Model file for the job. Use its own axes, mm. Face numbers are marked on the shaded views. A direction names the side the tool comes from. Coordinates: 2 decimals unless noted, no trailing zeros. Write each loop counter-clockwise with the first axis right and the second up, starting at its lowest first coordinate (ties: lowest second). Pieces come first, ordered by that corner, then holes. Notation, with made-up numbers: M 13.5,64.25 L 35.5,64.25 A18 ccw 35.5,96.25 Z; hole C 40,-12.5 d2. An arc over 180 degrees is marked long. One line per question, with ' | ' between items. Start each with the question number.
(1) Cut at A-A (y = -35). Write the cut outline in (x, z).
(2) Cut at B-B (z = 4). Write the cut outline in (x, y), plus the area to 3 significant figures.
(3) Flat gauge pins, fed straight in: pin 1 Ø8 at (y, z) = (-10, 1.5) entering from +X; pin 2 Ø3.5 at (x, z) = (11, 5) entering from +Y; pin 3 Ø5 at (y, z) = (-18, 22) entering from -X; pin 4 Ø4.5 at (y, z) = (-22.5, 2) entering from -X. Where does each tip first touch, or does it go through?
(4) Wall check: probe 1 along Y at (x, z) = (14.75, 7); probe 2 along Y at (x, z) = (8, 20); probe 3 along Z at (x, y) = (8, -33). Give the ranges that are in metal, low to high.
(5) Two-plate mould, pull along Z, no slides. Class the marked faces 1, 2 and 3: +Z half, -Z half, draft (parallel to the pull), parting line (faces both ways), or undercut.
(6) Tool access for the marked faces 4, 5, 6 and 7: list every direction of +Z, -Z, +X, -X, +Y, -Y with a clear straight run to the whole face (end or side of a thin tool).
(7) Cut at D-D (y = -9). Write the cut outline in (x, z).
(8) Cut at C-C (x = 11.75). Write the cut outline in (y, z).
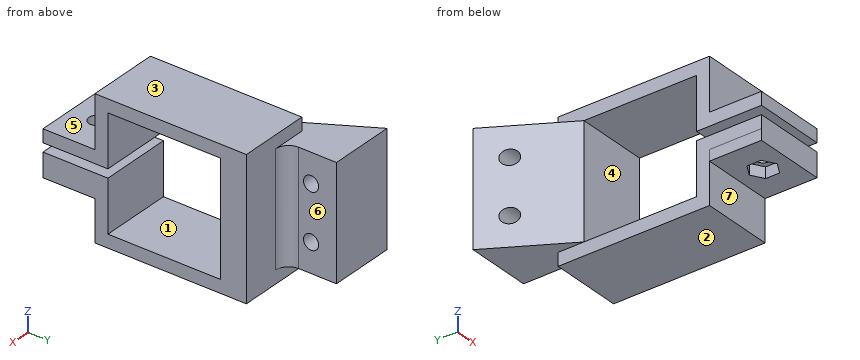
from build123d import *

# Parameters (mm, degrees)
BOSS_EXTRUDE1_DEPTH = 26
SKETCH3_R           = 1.75
CUT_EXTRUDE2_DEPTH  = 35.925597792
FILLET1_R           = 3
BOSS_EXTRUDE2_DEPTH = 16.626016
SKETCH5_R           = 1.8
CUT_EXTRUDE3_DEPTH  = 49.553315232
SKETCH6_W           = 16.626016361
SKETCH6_H           = 12
BOSS_EXTRUDE3_DEPTH = 2.5


with BuildPart() as part:
    # Sketch1 → Boss-Extrude1 (new body)
    with BuildSketch(Plane.XY):
        Polygon((0, 0), (-10.247967278, 17.75), (4.876016361, 17.75), (4.876016361, 6), (16.626016361, 6), (16.626016361, 0), align=None)
    extrude(amount=BOSS_EXTRUDE1_DEPTH)

    # Sketch3 → Cut-Extrude2 (cut, through all)
    with BuildSketch(Plane(origin=(4.876016361, 0, 0), x_dir=(0, 0, -1), z_dir=(1, 0, 0))):
        with Locations(Location((-19.25, 11.875, 0), (0, 0, 90))):
            Circle(SKETCH3_R)
        with Locations(Location((-6.75, 11.875, 0), (0, 0, 90))):
            Circle(SKETCH3_R)
    extrude(amount=-CUT_EXTRUDE2_DEPTH, mode=Mode.SUBTRACT)

    # Fillet1
    fillet1_edges = [part.edges().sort_by_distance(p)[0] for p in [
        (4.876016361, 6, 13),
    ]]
    fillet(fillet1_edges, radius=FILLET1_R)

    # Sketch4 → Boss-Extrude2 (add)
    with BuildSketch(Plane(origin=(16.626016361, 0, 0), x_dir=(0, 0, -1), z_dir=(1, 0, 0))):
        Polygon((-26, 6), (-29, 6), (-29, -29), (-17, -29), (-17, -41), (-14, -41), (-14, -26), (-26, -26), (-26, 0), align=None)
    boss_extrude2 = extrude(amount=-BOSS_EXTRUDE2_DEPTH)

    # Mirror1: Boss-Extrude2 across plane
    add(boss_extrude2.mirror(Plane(origin=(0, 0, 13), x_dir=(1, 0, 0), z_dir=(0, 0, -1))))

    # Sketch5 → Cut-Extrude3 (cut, through all)
    with BuildSketch(Plane.XY.offset(17)):
        with Locations(Location((8.31300818, -35, 0), (0, 0, 270))):
            Circle(SKETCH5_R)
    extrude(amount=-CUT_EXTRUDE3_DEPTH, mode=Mode.SUBTRACT)

    # Sketch6 → Boss-Extrude3 (add)
    with BuildSketch(Plane(origin=(0, 0, 9), x_dir=(-1, 0, 0), z_dir=(0, 0, -1))):
        with Locations((-8.313008181, -35)):
            Rectangle(SKETCH6_W, SKETCH6_H)
        Polygon((-5.51300818, -33.383419246), (-8.31300818, -31.766838493), (-11.11300818, -33.383419246), (-11.11300818, -36.616580754), (-8.31300818, -38.233161507), (-5.51300818, -36.616580754), align=None, mode=Mode.SUBTRACT)
    extrude(amount=BOSS_EXTRUDE3_DEPTH)


solid = part.part
Filled in:
1) outline: M 0,6.5 L 5.51,6.5 L 5.51,9 L 6.51,9 L 6.51,12 L 0,12 Z; M 0,14 L 6.51,14 L 6.51,17 L 0,17 Z; M 10.11,9 L 11.11,9 L 11.11,6.5 L 16.63,6.5 L 16.63,12 L 10.11,12 Z; M 10.11,14 L 16.63,14 L 16.63,17 L 10.11,17 Z
2) outline: M -10.25,17.75 L 0,0 L 16.63,0 L 16.63,6 L 7.88,6 A3 cw 4.88,9 L 4.88,17.75 Z; M 0,-29 L 16.63,-29 L 16.63,-26 L 0,-26 Z | area: 300 mm²
3) pin 1: x = 16.63 | pin 2: y = 6 | pin 3: through | pin 4: x = 0
4) probe 1: -41 to -26, 0 to 6 | probe 2: -29 to -26, 0 to 6 | probe 3: 9 to 12, 14 to 17
5) face 1: undercut | face 2: -Z half | face 3: +Z half
6) face 4: +X, -X | face 5: +Z, +X, -X, -Y | face 6: +Z, -Z, +X, +Y | face 7: -Z, +X, -X, -Y
7) outline: M 0,-3 L 16.63,-3 L 16.63,0 L 0,0 Z; M 0,26 L 16.63,26 L 16.63,29 L 0,29 Z
8) outline: M -41,6.5 L -29,6.5 L -29,-3 L 6,-3 L 6,29 L -29,29 L -29,17 L -41,17 L -41,14 L -26,14 L -26,26 L 0,26 L 0,0 L -26,0 L -26,12 L -41,12 Z
